Autodesk Fusion 360 part; units mm, degrees
sketch "Sketch1" plane through (0, 0, 0) normal (0, 0, 1) x (1, 0, 0)
  line L0 (-100, 60) -> (100, 60)
  line L1 (100, 60) -> (100, -60)
  line L2 (100, -60) -> (-100, -60)
  line L3 (-100, -60) -> (-100, 60)
  line L4 (-100, 60) -> (100, -60) construction
  line L5 (100, 60) -> (-100, -60) construction
extrude "Extrude1" add sketch "Sketch1" along normal blind 20
sketch "Sketch2" plane through (0, 0, 20) normal (0, 0, 1) x (-1, 0, 0)
  line L0 (100, 60) -> (-100, 60)
  line L1 (-100, 60) -> (-100, -60)
  line L2 (-100, -60) -> (100, -60)
  line L3 (100, -60) -> (100, 60)
  line L4 (80, -40) -> (-80, -40)
  line L5 (-80, -40) -> (-80, 40)
  line L6 (-80, 40) -> (80, 40)
  line L7 (80, 40) -> (80, -40)
  line L8 (80, -40) -> (-80, 40) construction
  line L9 (-80, -40) -> (80, 40) construction
hole "Hole1" at (-80, 40, 20) at (-80, -40, 20) at (80, 40, 20) at (80, -40, 20) direction (0, 0, -1) diameter 18.022 depth 20 tip angle 118
Can you work these out from the model? Positions are in its coordinate system, mm. Round coordinates to 2 decimals unless told otherwise and drop trailing zeros. Loops run counter-clockwise (first coordinate to the right, second up) from the corner with the lowest first, then second, coordinate; pieces in that order, holes last. Notation, with made-up numbers: (65, 25.25) - (85, 25.25) arc R7 cw to (85, 37.25) - close; hole circle Ø7 at (28, 62.5). An arc over 180 degrees is marked (long way). Use CSV: the item, a comma, the result in double quotes. Start each with the question number.
1) If we section it at C-C on y = -40: Write out the boundary of the cut face in (x, z), plus the area to 3 significant figures.
2) We'd pull the mould along X, two halves only. Please class faces 1 (the cylindrical face through (-72.006, -44.158, 9.86)), 2 (the flat face through (-1, 60, 10)), 3 (the flat face through (-100, -1, 10)), 4 (the cylindrical face through (87.994, 35.842, 9.86)): released by +X, released by -X, zero draft, split by the parting line, or undercut.
3) If we section it at A-A on x = 80: Write out the boundary of the cut face in (y, z), plus the area to 3 significant figures.
4) If we section it at B-B on z = 17.75: Write out the boundary of the cut face in (x, y), plus the area to 3 significant figures.
5) Please list where these lines run through material, in increasing order: probe 1 along X at (y, z) = (40, 11.75); probe 2 along Y at (x, z) = (80, 14.75); probe 3 along Y at (x, z) = (85.5, 16.75). Write a range as [from, to].
Geometry results:
1,outline,"(-100, 0) - (-89.01, 0) - (-89.01, 20) - (-100, 20) - close; (-70.99, 0) - (70.99, 0) - (70.99, 20) - (-70.99, 20) - close; (89.01, 0) - (100, 0) - (100, 20) - (89.01, 20) - close"
1,area,"3,280 mm2"
2,face 1,"undercut"
2,face 2,"zero draft"
2,face 3,"released by -X"
2,face 4,"undercut"
3,outline,"(-60, 0) - (-49.01, 0) - (-49.01, 20) - (-60, 20) - close; (-30.99, 0) - (30.99, 0) - (30.99, 20) - (-30.99, 20) - close; (49.01, 0) - (60, 0) - (60, 20) - (49.01, 20) - close"
3,area,"1,680 mm2"
4,outline,"(-100, -60) - (100, -60) - (100, 60) - (-100, 60) - close; hole circle Ø18.02 at (-80, -40); hole circle Ø18.02 at (-80, 40); hole circle Ø18.02 at (80, -40); hole circle Ø18.02 at (80, 40)"
4,area,"23,000 mm2"
5,probe 1,"x = [-100, -89.01], [-70.99, 70.99], [89.01, 100]"
5,probe 2,"y = [-60, -49.01], [-30.99, 30.99], [49.01, 60]"
5,probe 3,"y = [-60, -47.14], [-32.86, 32.86], [47.14, 60]"
